Can you work these out from the model? Positions are in its coordinate system, mm. A direction names the side the tool comes from. Give positions to 0.01 mm unless a question says otherwise; leave off trailing zeros. Order: outer loops, then holes, each group sorted by start corner. A loop starts at its lowest first (then second) coordinate and runs counter-clockwise, first axis right, second up. Notation, with made-up numbers: (12.25, -12) - (61.25, -12) arc R28 cw to (61.25, 18) - close; hole circle Ø10 at (76, 30). An arc over 180 degrees is marked (long way). One line per question, with ' | ' between items.
```python
from build123d import *

# Parameters (mm, degrees)
SKETCH1_R               = 101.6
SKETCH1_R_2             = 95.25
BOSS_EXTRUDE1_DEPTH     = 25.4
SKETCH2_R               = 3.175
CUT_EXTRUDE1_DEPTH      = 102.6
CUT_EXTRUDE1_DEPTH_BACK = 102.6
SKETCH5_R               = 101.6
SKETCH5_R_2             = 98.425
BOSS_EXTRUDE2_DEPTH     = 146.05
SKETCH9_R               = 2.1
CUT_EXTRUDE5_DEPTH      = 204.2000001
SKETCH10_R              = 101.6
CUT_EXTRUDE6_DEPTH      = 120.65


with BuildPart() as part:
    # Sketch1 → Boss-Extrude1 (new body)
    with BuildSketch(Plane(origin=(0, 0, 0), x_dir=(1, 0, 0), z_dir=(0, 1, 0))):
        Circle(SKETCH1_R)
        Circle(SKETCH1_R_2, mode=Mode.SUBTRACT)
    extrude(amount=BOSS_EXTRUDE1_DEPTH)

    # Sketch2 → Cut-Extrude1 (cut, two sides)
    with BuildSketch(Plane.XY) as cut_extrude1_sk:
        with Locations((0, 12.7)):
            Circle(SKETCH2_R)
    extrude(amount=CUT_EXTRUDE1_DEPTH, mode=Mode.SUBTRACT)
    extrude(cut_extrude1_sk.sketch, amount=-CUT_EXTRUDE1_DEPTH_BACK, mode=Mode.SUBTRACT)

    # Sketch5 → Boss-Extrude2 (add)
    with BuildSketch(Plane(origin=(0, 25.4, 0), x_dir=(1, 0, 0), z_dir=(0, 1, 0))):
        Circle(SKETCH5_R)
        Circle(SKETCH5_R_2, mode=Mode.SUBTRACT)
    extrude(amount=BOSS_EXTRUDE2_DEPTH)

    # Sketch9 → Cut-Extrude5 (cut, through all)
    with BuildSketch(Plane.XY.offset(101.6)):
        with Locations((-85.075, 156.8)):
            Circle(SKETCH9_R)
    extrude(amount=-CUT_EXTRUDE5_DEPTH, mode=Mode.SUBTRACT)

    # Sketch10 → Cut-Extrude6 (cut)
    with BuildSketch(Plane(origin=(0, 171.45, 0), x_dir=(1, 0, 0), z_dir=(0, 1, 0))):
        Circle(SKETCH10_R)
    extrude(amount=-CUT_EXTRUDE6_DEPTH, mode=Mode.SUBTRACT)


solid = part.part
```
(1) Imagine slicing it at B-B (x = -71). List the corners of the cut face in (y, z) for me, and give its area (3 significant figures).
Answer below:
outline: (0, -72.67) - (50.8, -72.67) - (50.8, -68.17) - (25.4, -68.17) - (25.4, -63.49) - (0, -63.49) - close; (0, 63.49) - (25.4, 63.49) - (25.4, 68.17) - (50.8, 68.17) - (50.8, 72.67) - (0, 72.67) - close | area: 695 mm^2
(2) Imagine slicing it at A-A (z = 0). List the corners of the cut face in (x, y) for me (3 decimals), and give its area (3 significant figures).
Answer below:
outline: (-101.6, 0) - (-95.25, 0) - (-95.25, 25.4) - (-98.425, 25.4) - (-98.425, 50.8) - (-101.6, 50.8) - close; (95.25, 0) - (101.6, 0) - (101.6, 50.8) - (98.425, 50.8) - (98.425, 25.4) - (95.25, 25.4) - close | area: 484 mm^2
(3) Imagine slicing it at D-D (x = 0.5). List the corners of the cut face in (y, z) for me.
Answer below:
outline: (0, -101.6) - (9.56, -101.6) - (9.56, -95.25) - (0, -95.25) - close; (0, 95.25) - (9.56, 95.25) - (9.56, 101.6) - (0, 101.6) - close; (15.84, -101.6) - (50.8, -101.6) - (50.8, -98.42) - (25.4, -98.42) - (25.4, -95.25) - (15.84, -95.25) - close; (15.84, 95.25) - (25.4, 95.25) - (25.4, 98.42) - (50.8, 98.42) - (50.8, 101.6) - (15.84, 101.6) - close
(4) On a 3-axis mill with a long thin cutter (end or side, diameter ignored), from which of +Z, -Z, +X, -X, +Y, -Y can I reach the whole of each face in a straight line? I mean faces 1 (the face through (1.5, 9.9, 98.4)), 2 (the face through (-51, 25.4, -81)). Say none if no direction works.
Answer below:
face 1: +Z, -Z | face 2: +Y
(5) If we mould it in two halves opening along X, with no side actions, what happens to faces 3 (the face through (-22.025, 25.044, 99.184)), 4 (the face through (93.88, 37.92, -29.56)), 5 (the face through (-83.3, 50.8, -53.2))? For each: released by +X, released by -X, zero draft, split by the parting line, or undercut.
Answer below:
face 3: split by the parting line | face 4: undercut | face 5: zero draft
(6) If I drill on line 1 (X direction, y = 18.25, z = 0); line 2 (Z direction, x = 1.5, y = 48.5); line 3 (X direction, y = 44.5, z = 0) (3 decimals), over which ranges is the centre line in solid material (lowest first)?
Answer below:
line 1: -101.6 to -95.25, 95.25 to 101.6 | line 2: -101.59 to -98.41, 98.41 to 101.59 | line 3: -101.6 to -98.425, 98.425 to 101.6
(7) Will these pins go through, and if not, where does the flat tip stop? pin 1 (5 mm diameter, centred on x = 35, y = 37, fed in from +Z); pin 2 (10 mm diameter, centred on x = 80, z = -30, fed in from +Y); pin 3 (5 mm diameter, centred on x = -30, y = 35, fed in from +Z); pin 4 (3 mm diameter, centred on y = 32, z = -51.5, fed in from +X).
Answer below:
pin 1: z = 96.26 | pin 2: through | pin 3: z = 97.81 | pin 4: x = 88.45
(8) Imagine slicing it at C-C (y = 12.7). List the corners of the cut face in (x, z) for me (3 decimals), and give its area (3 significant figures).
Answer below:
outline: (-3.175, -101.55) - (-3.175, -95.197) arc R95.25 cw to (-3.175, 95.197) - (-3.175, 101.55) arc R101.6 ccw to start; (3.175, -101.55) arc R101.6 ccw to (3.175, 101.55) - (3.175, 95.197) arc R95.25 cw to (3.175, -95.197) - close | area: 3,850 mm^2
